```python
from build123d import *

# Parameters (mm, degrees)
SKETCH_1_W          = 135
SKETCH_1_H          = 73
SKETCH_1_R          = 1.75
EXTRUDE_1_DEPTH     = 1.5
EXTRUDE_2_DEPTH     = 1.5
SKETCH_3_R          = 1.75
CUT_EXTRUDE_1_DEPTH = 10
SKETCH_4_W          = 41.774979177
SKETCH_4_H          = 174.552922684
SKETCH_4_W_2        = 25.198535703
SKETCH_4_H_2        = 178.613265212
SKETCH_4_W_3        = 80
SKETCH_4_H_3        = 12.9239929
CUT_EXTRUDE_2_DEPTH = 10
SKETCH_5_W          = 120
SKETCH_5_H          = 1.5
EXTRUDE_3_DEPTH     = 20
SKETCH_6_R          = 1.75
CUT_EXTRUDE_3_DEPTH = 20
CHAMFER_1_SIZE      = 1.25


with BuildPart() as part:
    # Эскиз1 → Вытянуть1 (new body)
    with BuildSketch(Plane.XY):
        with Locations((67.5, 36.5)):
            Rectangle(SKETCH_1_W, SKETCH_1_H)
        with Locations((118, 55)):
            Circle(SKETCH_1_R, mode=Mode.SUBTRACT)
        with Locations((29, 60)):
            Circle(SKETCH_1_R, mode=Mode.SUBTRACT)
        with Locations((67, 8)):
            Circle(SKETCH_1_R, mode=Mode.SUBTRACT)
    extrude(amount=EXTRUDE_1_DEPTH)

    # Эскиз2 → Вытянуть2 (add)
    with BuildSketch(Plane(origin=(0, 0, 0), x_dir=(-1, 0, 0), z_dir=(0, 0, -1))):
        Polygon((-135, 0), (-135, 73), (-137.5, 73), (-137.5, -77), (12.5, -77), (12.5, 73), (0, 73), (0, 0), align=None)
    extrude(amount=-EXTRUDE_2_DEPTH)

    # Эскиз3 → Вырез-Вытянуть1 (cut)
    with BuildSketch(Plane(origin=(0, 0, 0), x_dir=(-1, 0, 0), z_dir=(0, 0, -1))):
        with Locations((-109, 58)):
            Circle(SKETCH_3_R)
        with Locations((-109, -72)):
            Circle(SKETCH_3_R)
        with Locations((-19, -72)):
            Circle(SKETCH_3_R)
        with Locations((-19, 58)):
            Circle(SKETCH_3_R)
    extrude(amount=-CUT_EXTRUDE_1_DEPTH, mode=Mode.SUBTRACT)

    # Эскиз4 → Вырез-Вытянуть2 (cut)
    with BuildSketch(Plane(origin=(0, 0, 0), x_dir=(-1, 0, 0), z_dir=(0, 0, -1))):
        with Locations((17.887489589, -5.455920086)):
            Rectangle(SKETCH_4_W, SKETCH_4_H)
        with Locations((-135.599267852, -7.48609135)):
            Rectangle(SKETCH_4_W_2, SKETCH_4_H_2)
        with Locations((-64, 71.46199645)):
            Rectangle(SKETCH_4_W_3, SKETCH_4_H_3)
    extrude(amount=-CUT_EXTRUDE_2_DEPTH, mode=Mode.SUBTRACT)

    # Эскиз5 → Вытянуть3 (add)
    with BuildSketch(Plane.XZ.offset(77)):
        with Locations((63, 0.75)):
            Rectangle(SKETCH_5_W, SKETCH_5_H)
    extrude(amount=EXTRUDE_3_DEPTH)

    # Эскиз6 → Вырез-Вытянуть3 (cut)
    with BuildSketch(Plane(origin=(0, 0, 0), x_dir=(-1, 0, 0), z_dir=(0, 0, -1))):
        with Locations((-8, -92)):
            Circle(SKETCH_6_R)
    extrude(amount=-CUT_EXTRUDE_3_DEPTH, mode=Mode.SUBTRACT)

    # Фаска1
    chamfer_1_edges = [part.edges().sort_by_distance(p)[0] for p in [
        (110.75, 58, 0),
        (110.75, -72, 0),
        (20.75, -72, 0),
        (20.75, 58, 0),
    ]]
    chamfer(chamfer_1_edges, length=CHAMFER_1_SIZE)


solid = part.part
```
Can you work these out from the model? Positions are in its coordinate system, mm. Round coordinates to 2 decimals unless told otherwise and drop trailing zeros. Loops run counter-clockwise (first coordinate to the right, second up) from the corner with the lowest first, then second, coordinate; pieces in that order, holes last.
Item 1: Suppose I cut it at C-C, the plane y = -72. Write out the boundary of the cut face in (x, z).
Item 2: Suppose I cut it at A-A, the plane x = 19. Write out the boundary of the cut face in (y, z).
Item 3: Suppose I cut it at B-B, the plane z = 0.7. State how many separate pieces and enclosed holes the cut face has, then the cut area to 3 significant figures.
Item 4: If we mould it in two halves opening along X, with no side actions, what happens to faces 1 (the conical face through (19, 60, 1)), 2 (the flat face through (62, -11, 1.5))? For each: +X half, -X half, draft (parallel to the pull), parting line (faces both ways), or undercut.
Item 5: Will this pin go through, and if not, where does the flat tip stop? pin 1 Ø5.5 at (x, y) = (19, -72) entering from -Z.
Item 6: Suppose I cut it at D-D, the plane y = 8. Write out the boundary of the cut face in (x, z), then the cut area to 3 significant figures.
Item 7: Please list where these lines run through material, in increasing order: L1, parallel to Y at x = 109, z = 1.35; L2, parallel to X at y = -72, z = 1.3; L3, parallel to X at y = -92, z = 0.6.
Reported:
1. outline: (3, 0) - (16, 0) - (17.25, 1.25) - (17.25, 1.5) - (3, 1.5) - close; (20.75, 1.25) - (22, 0) - (106, 0) - (107.25, 1.25) - (107.25, 1.5) - (20.75, 1.5) - close; (110.75, 1.25) - (112, 0) - (123, 0) - (123, 1.5) - (110.75, 1.5) - close
2. outline: (-97, 0) - (-75, 0) - (-73.75, 1.25) - (-73.75, 1.5) - (-97, 1.5) - close; (-70.25, 1.25) - (-69, 0) - (55, 0) - (56.25, 1.25) - (56.25, 1.5) - (-70.25, 1.5) - close; (59.75, 1.25) - (61, 0) - (73, 0) - (73, 1.5) - (59.75, 1.5) - close
3. separate pieces: 1
3. enclosed holes: 8
3. area: 19,700 mm2
4. face 1: undercut
4. face 2: draft
5. pin 1: stops at z = 0.25
6. outline: (3, 0) - (65.25, 0) - (65.25, 1.5) - (3, 1.5) - close; (68.75, 0) - (123, 0) - (123, 1.5) - (68.75, 1.5) - close
6. area: 175 mm2
7. L1: y = -97 to -73.75, -70.25 to 56.25, 59.75 to 73
7. L2: x = 3 to 17.25, 20.75 to 107.25, 110.75 to 123
7. L3: x = 3 to 6.25, 9.75 to 123
